For this review, take the finished solid that the model builds, in its own axes (mm). Coordinates: 2 decimals unless noted, no trailing zeros. Loops run counter-clockwise (first coordinate to the right, second up) from the corner with the lowest first, then second, coordinate; pieces in that order, holes last.
1. Take a section at C-C, the plane y = 1.5. State the section outline as (x, z) points, then the cut area to 3 significant figures.
2. Take a section at A-A, the plane z = 2.45. State the section outline as (x, y) points, then the cut area to 3 significant figures.
3. Take a section at D-D, the plane y = -39. State the section outline as (x, z) points.
4. Take a section at B-B, the plane x = 40.5. State the section outline as (y, z) points, then the cut area to 3 significant figures.
5. Mouldability with a two-part tool opening along X and no side actions: class faces 1 (the face through (43, 0, 2)), 2 (the face through (119.995, 1.08, 1.479)), 3 (the face through (9.654, -41.08, 1.479)) as pulls with the +X half, pulls with the -X half, needs draft (parallel to the pull), parting line crosses it, or undercut.
6. Clearance check with flat-ended pins moving along their axes: P1, Ø12.5, axis at x = 42, y = 2, coming from the +Z side; P2, Ø1, axis at x = 68, z = 1, coming from the -Y side; P3, Ø1.1, axis at x = 53, z = 2.5, coming from the +Y side. State where each tip first meets the part, or that it passes through.
7. To check wall thickness, follow probe 1 along Z at (x, y) = (54.5, -3); probe 2 along Y at (x, z) = (23, 2.3); probe 3 along X at (y, z) = (0, 1.6). State the ranges of each line that lie inside material, in increasing order.
Autodesk Inventor part; units mm, degrees
ref_plane "YZ Plane" through (0, 0, 0) normal (1, 0, 0) x (0, 1, 0)
ref_plane "XZ Plane" through (0, 0, 0) normal (0, 1, 0) x (-1, 0, 0)
ref_plane "XY Plane" through (0, 0, 0) normal (0, 0, 1) x (1, 0, 0)
sketch "Sketch3" plane through (0, 0, 0) normal (0, 0, 1) x (1, 0, 0)
  line L0 (-124.5182, 0) -> (335.753, 0)
  line L1 (0, -1648.3682) -> (0, 1648.3682)
  line L2 (-58.7652, -57.1704) -> (105.7311, -56.7534) construction
  line L3 (17.7382, 55.0824) -> (1.3397, 26.6795)
  line L4 (17.7382, -55.0824) -> (1.3397, -26.6795)
  line L5 (20, -59) -> (52.7968, -59) construction
  arc A0 (23.8789, 59.7598) -> (17.7382, 55.0824) centre (26.3984, 50.0824) ccw
  arc A1 (17.7382, -55.0824) -> (23.8789, -59.7598) centre (26.3984, -50.0824) ccw
  line L6 (0, 21.6795) -> (0, -21.6795)
  arc A2 (96.0371, -71.9505) -> (96.0371, 71.9505) centre (0, 0) ccw
  line L7 (96.0371, 71.9505) -> (96.0371, -71.9505) construction
  arc A3 (96.0371, 71.9505) -> (23.8789, 59.7598) centre (270, -1177.4058) ccw
  arc A4 (23.8789, -59.7598) -> (96.0371, -71.9505) centre (270, 1177.4058) ccw
  arc A5 (1.3397, 26.6795) -> (0, 21.6795) centre (10, 21.6795) ccw
  arc A6 (0, -21.6795) -> (1.3397, -26.6795) centre (10, -21.6795) ccw
  point P0 (0, 24.359)
  point P1 (0, -24.359)
  point P2 (0, -24.359)
  dimension "d8" = 40
  dimension "d9" = 120
  dimension "d10" = 10
  dimension "d11" = 10
  dimension "d13" = 120
  dimension "d15" = 48.718
  dimension "d16" = 30.7234
  dimension "d17" = 30.7234
  dimension "d18" = 100.1648
  dimension "d19" = 270
  dimension "d20" = 1261.4097
  dimension "d21" = 10
  dimension "d24" = 143.901
extrude "Extrusion1" add sketch "Sketch3" along normal blind 3
sketch "Sketch4" plane through (0, 0, 3) normal (0, 0, 1) x (1, 0, 0)
  line L0 (15.466, -12.5) -> (70.466, -12.5)
  line L1 (70.466, -12.5) -> (70.466, 12.5)
  line L2 (70.466, 12.5) -> (15.466, 12.5)
  line L3 (15.466, 12.5) -> (15.466, -12.5)
  line L4 (15.466, -12.5) -> (70.466, 12.5) construction
  line L5 (70.466, -12.5) -> (15.466, 12.5) construction
  point P0 (0, 0)
  point P1 (42.966, 0)
  dimension "d31" = 55
  dimension "d32" = 25
extrude "Extrusion2" cut sketch "Sketch4" against normal blind 1
equation "\"d9\" = d7"
equation "\"d11\" = d10"
equation "\"BendRadius\" = Thickness"
equation "\"BendReliefWidth\" = Thickness"
equation "\"BendReliefDepth\" = 0.5 * Thickness"
equation "\"CornerReliefSize\" = 4 * Thickness"
equation "\"MinimumRemnant\" = 2 * Thickness"
equation "\"TransitionRadius\" = BendRadius"
equation "\"JacobiRadiusSize\" = BendRadius"
equation "\"GapSize\" = Thickness"
properties part number "Handle bars holder plates"
Results list:
1. outline: (0, 0) - (119.99, 0) - (119.99, 3) - (70.47, 3) - (70.47, 2) - (15.47, 2) - (15.47, 3) - (0, 3) - close
1. area: 305 mm2
2. outline: (0, -21.68) arc R10 ccw to (1.34, -26.68) - (17.74, -55.08) arc R10 ccw to (23.88, -59.76) arc R1261.38 ccw to (96.04, -71.95) arc R120 ccw to (96.04, 71.95) arc R1261.44 ccw to (23.88, 59.76) arc R10 ccw to (17.74, 55.08) - (1.34, 26.68) arc R10 ccw to (0, 21.68) - close; hole (15.47, -12.5) - (70.47, -12.5) - (70.47, 12.5) - (15.47, 12.5) - close
2. area: 12,700 mm2
3. outline: (8.45, 0) - (113.49, 0) - (113.49, 3) - (8.45, 3) - close
4. outline: (-62.95, 0) - (62.95, 0) - (62.95, 3) - (12.5, 3) - (12.5, 2) - (-12.5, 2) - (-12.5, 3) - (-62.95, 3) - close
4. area: 353 mm2
5. face 1: undercut
5. face 2: pulls with the +X half
5. face 3: pulls with the -X half
6. P1: stops at z = 2
6. P2: stops at y = -67.81
6. P3: stops at y = 65.29
7. probe 1: z = 0 to 2
7. probe 2: y = -59.49 to -12.5, 12.5 to 59.49
7. probe 3: x = 0 to 120
